The listing builds one solid part. Answer for the finished solid, in the listing's coordinates (mm). Face numbers are marked on the shaded views. Round coordinates to 2 decimals unless told otherwise and drop trailing zeros. Write each loop counter-clockwise with the first axis right and the second up, starting at its lowest first coordinate (ties: lowest second). Pieces come first, ordered by that corner, then holes.
Item 1: Find the intervals of material crossed by probe 1 along Z at (x, y) = (0.6, 85); probe 2 along Y at (x, z) = (4.1, 0), in increasing order.
Item 2: Each of these flat-tipped pins is pushed along its axis until it touches: pin 1 (2.5 mm diameter, centred on x = 2, z = -77, fed in from +Y); pin 2 (3 mm diameter, centred on x = 4.5, y = 15, fed in from -Z) (3 decimals); pin 3 (1.5 mm diameter, centred on x = 1, y = 78.5, fed in from +Z). Where does it stop, or does it pass through?
Item 3: Find section C-C on z = -6. Give the vertices of the cut face in (x, y), then the cut area to 3 significant figures.
Item 4: For a pull along Y with two mould halves and no side action, classify the marked faces 1 and 2 as +Y half, -Y half, draft (parallel to the pull), parting line (faces both ways), or undercut.
Item 5: Find section A-A on x = 1.6. Give the vertices of the cut face in (y, z).
Item 6: Find section D-D on y = -18. Give the vertices of the cut face in (x, z), then the cut area to 3 significant figures.
Item 7: Find section B-B on y = -38.5. Give the vertices of the cut face in (x, z).
```python
from build123d import *

# Parameters (mm, degrees)
SKETCH_1_R      = 75
SKETCH_1_R_2    = 1.5
EXTRUDE_1_DEPTH = 3
SKETCH_2_R      = 75
SKETCH_2_R_2    = 60
EXTRUDE_2_DEPTH = 3


with BuildPart() as part:
    # Эскиз1 → Бобышка-Вытянуть1 (new body)
    # profile 1 of 5: a face of its own
    with BuildSketch(Plane(origin=(0, 0, 0), x_dir=(0, 0, -1), z_dir=(1, 0, 0))):
        Circle(SKETCH_1_R)
    # profile 2 of 5: a face of its own
    with BuildSketch(Plane(origin=(0, 0, 0), x_dir=(0, 0, -1), z_dir=(1, 0, 0))):
        with BuildLine():
            ThreePointArc((-8.5, 74.516776635), (0, 75), (8.5, 74.516776635))
            Line((8.5, 74.516776635), (8.5, 85))
            ThreePointArc((8.5, 85), (0, 93.5), (-8.5, 85))
            Line((-8.5, 85), (-8.5, 74.516776635))
        make_face()
        with BuildLine():
            ThreePointArc((0, 83.5), (-1.060660172, 86.060660172), (1.5, 85))
            ThreePointArc((1.5, 85), (1.060660172, 83.939339828), (0, 83.5))
        make_face(mode=Mode.SUBTRACT)
    # profile 3 of 5: a face of its own
    with BuildSketch(Plane(origin=(0, 0, 0), x_dir=(0, 0, -1), z_dir=(1, 0, 0))):
        with BuildLine():
            ThreePointArc((85, -8.5), (93.5, 0), (85, 8.5))
            Line((85, 8.5), (74.516776635, 8.5))
            ThreePointArc((74.516776635, 8.5), (74.879096708, 4.256862249), (75, 0))
            ThreePointArc((75, 0), (74.879096708, -4.256862249), (74.516776635, -8.5))
            Line((74.516776635, -8.5), (85, -8.5))
        make_face()
        with BuildLine():
            ThreePointArc((83.5, 0), (85, 1.5), (86.5, 0))
            ThreePointArc((86.5, 0), (85, -1.5), (83.5, 0))
        make_face(mode=Mode.SUBTRACT)
    # profile 4 of 5: a face of its own
    with BuildSketch(Plane(origin=(0, 0, 0), x_dir=(0, 0, -1), z_dir=(1, 0, 0))):
        with BuildLine():
            Line((8.5, -85), (8.5, -74.516776635))
            ThreePointArc((8.5, -74.516776635), (0, -75), (-8.5, -74.516776635))
            Line((-8.5, -74.516776635), (-8.5, -85))
            ThreePointArc((-8.5, -85), (0, -93.5), (8.5, -85))
        make_face()
        with BuildLine():
            ThreePointArc((0, -83.5), (1.060660172, -83.939339828), (1.5, -85))
            ThreePointArc((1.5, -85), (-1.060660172, -86.060660172), (0, -83.5))
        make_face(mode=Mode.SUBTRACT)
    # profile 5 of 5: a face of its own
    with BuildSketch(Plane(origin=(0, 0, 0), x_dir=(0, 0, -1), z_dir=(1, 0, 0))):
        with BuildLine():
            ThreePointArc((-74.516776635, -8.5), (-75, 0), (-74.516776635, 8.5))
            Line((-74.516776635, 8.5), (-85, 8.5))
            ThreePointArc((-85, 8.5), (-93.5, 0), (-85, -8.5))
            Line((-85, -8.5), (-74.516776635, -8.5))
        make_face()
        with Locations((-85, 0)):
            Circle(SKETCH_1_R_2, mode=Mode.SUBTRACT)
    extrude(amount=EXTRUDE_1_DEPTH)

    # Эскиз2 → Бобышка-Вытянуть2 (add)
    with BuildSketch(Plane(origin=(3, 0, 0), x_dir=(0, 0, -1), z_dir=(1, 0, 0))):
        with Locations(Location((0, 0, 0), (0, 0, 173.492496408))):
            Circle(SKETCH_2_R)
        Circle(SKETCH_2_R_2, mode=Mode.SUBTRACT)
    extrude(amount=EXTRUDE_2_DEPTH)


solid = part.part
```
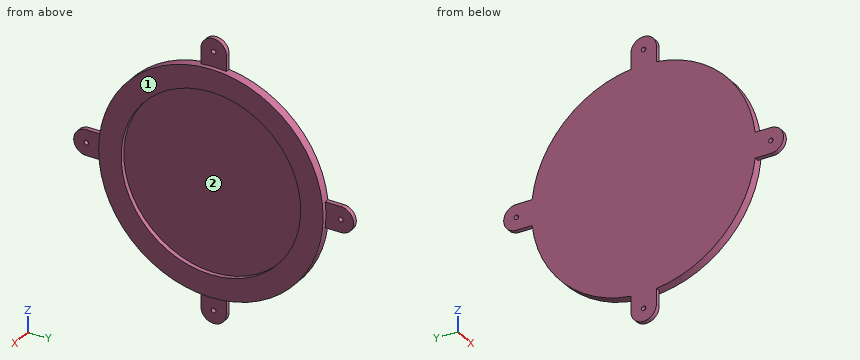
Check values:
1. probe 1: z = -8.5 to -1.5, 1.5 to 8.5
1. probe 2: y = -75 to -60, 60 to 75
2. pin 1: stops at y = 8.5
2. pin 2: stops at z = -73.775
2. pin 3: stops at z = 8.5
3. outline: (0, -91.02) - (3, -91.02) - (3, -74.76) - (6, -74.76) - (6, -59.7) - (3, -59.7) - (3, 59.7) - (6, 59.7) - (6, 74.76) - (3, 74.76) - (3, 91.02) - (0, 91.02) - close
3. area: 636 mm2
4. face 1: draft
4. face 2: undercut
5. outline: (-85, -8.5) - (-74.52, -8.5) arc R75 ccw to (-8.5, -74.52) - (-8.5, -85) arc R8.5 ccw to (8.5, -85) - (8.5, -74.52) arc R75 ccw to (74.52, -8.5) - (85, -8.5) arc R8.5 ccw to (85, 8.5) - (74.52, 8.5) arc R75 ccw to (8.5, 74.52) - (8.5, 85) arc R8.5 ccw to (-8.5, 85) - (-8.5, 74.52) arc R75 ccw to (-74.52, 8.5) - (-85, 8.5) arc R8.5 ccw to start; hole circle Ø3 at (-85, 0); hole circle Ø3 at (0, -85); hole circle Ø3 at (0, 85); hole circle Ø3 at (85, 0)
6. outline: (0, -72.81) - (6, -72.81) - (6, -57.24) - (3, -57.24) - (3, 57.24) - (6, 57.24) - (6, 72.81) - (0, 72.81) - close
6. area: 530 mm2
7. outline: (0, -64.36) - (6, -64.36) - (6, -46.02) - (3, -46.02) - (3, 46.02) - (6, 46.02) - (6, 64.36) - (0, 64.36) - close
